```python
from build123d import *

# Parameters (mm, degrees)
F0_R     = 38.1
F1_DEPTH = 1778
F2_R     = 34.925
F3_DEPTH = 25.4
F4_R     = 34.925
F5_DEPTH = 25.4
F6_W     = 25.4
F6_H     = 25.4
F7_DEPTH = 38.1
F8_W     = 25.4
F8_H     = 25.4
F9_DEPTH = 38.1
F10_R    = 5.08
F11_R    = 5.08


# Not quite as in the source:
# - a pattern or mirror of a feature is missing from the dataset's text; its kind, count and spacing are read off the source's solid


with BuildPart() as f1:
    # F0 (on Front) → F1 (new body)
    with BuildSketch(Plane.XZ):
        Circle(F0_R)
    extrude(amount=F1_DEPTH)

    # F2 (on face) → F3 (join)
    with BuildSketch(Plane.XZ.offset(1778)):
        Circle(F2_R)
    extrude(amount=F3_DEPTH)

    # F4 (on face) → F5 (join)
    with BuildSketch(Plane(origin=(0, 0, 0), x_dir=(-1, 0, 0), z_dir=(0, 1, 0))):
        Circle(F4_R)
    extrude(amount=F5_DEPTH)

    # F6 (on face) → F7 (join)
    with BuildSketch(Plane.XZ.offset(1803.4)):
        Rectangle(F6_W, F6_H)
    f7 = extrude(amount=F7_DEPTH)

    # F7_copies: F7 across plane
    add(f7.mirror(Plane.ZX.offset(-882.65)))

    # F8 (on face) → F9 (join)
    with BuildSketch(Plane(origin=(0, 25.4, 0), x_dir=(-1, 0, 0), z_dir=(0, 1, 0))):
        Rectangle(F8_W, F8_H)
    extrude(amount=F9_DEPTH)

    # F10
    f10_edges = [f1.edges().sort_by_distance(p)[0] for p in [
        (34.925, 25.4, 0),
    ]]
    fillet(f10_edges, radius=F10_R)

    # F11
    f11_edges = [f1.edges().sort_by_distance(p)[0] for p in [
        (-34.925, -1803.4, 0),
    ]]
    fillet(f11_edges, radius=F11_R)


solid = f1.part
```
Check sheet for the modelled part. Datum: model origin and axes. Units: mm. A direction names the side the tool comes from. Round coordinates to 2 decimals unless told otherwise and drop trailing zeros. Write each loop counter-clockwise with the first axis right and the second up, starting at its lowest first coordinate (ties: lowest second). Pieces come first, ordered by that corner, then holes. Notation, with made-up numbers: (67, -39) -> (117, -39) arc R28 cw to (117, -1) -> close; hole circle Ø1 at (-39.75, 30). An arc over 180 degrees is marked (long way). Put each result on its own line as item: value.
(1) Sectioned sample at B-B (x = 0). Enter the section's corners in (y, z) (3 decimals), plus the area to 3 significant figures.
Values found:
outline: (-1841.5, -12.7) -> (-1803.4, -12.7) -> (-1803.4, -29.845) arc R5.08 ccw to (-1798.32, -34.925) -> (-1778, -34.925) -> (-1778, -38.1) -> (0, -38.1) -> (0, -34.925) -> (20.32, -34.925) arc R5.08 ccw to (25.4, -29.845) -> (25.4, -12.7) -> (76.2, -12.7) -> (76.2, 12.7) -> (25.4, 12.7) -> (25.4, 29.845) arc R5.08 ccw to (20.32, 34.925) -> (0, 34.925) -> (0, 38.1) -> (-1778, 38.1) -> (-1778, 34.925) -> (-1798.32, 34.925) arc R5.08 ccw to (-1803.4, 29.845) -> (-1803.4, 12.7) -> (-1841.5, 12.7) -> close
area: 141,000 mm^2
(2) Material ranges on line 1 (Y direction, x = 30.5, z = -4); line 2 (Y direction, x = -5, z = 25.5); line 3 (Z direction, x = 14.5, y = -247.5), recorded low to high.
Values found:
line 1: y = -1803.32 to 25.32
line 2: y = -1803.4 to 25.4
line 3: z = -35.23 to 35.23
(3) Sectioned sample at A-A (z = 0). Enter the section's corners in (x, y) (3 decimals).
Values found:
outline: (-38.1, -1778) -> (-34.925, -1778) -> (-34.925, -1798.32) arc R5.08 ccw to (-29.845, -1803.4) -> (-12.7, -1803.4) -> (-12.7, -1841.5) -> (12.7, -1841.5) -> (12.7, -1803.4) -> (29.845, -1803.4) arc R5.08 ccw to (34.925, -1798.32) -> (34.925, -1778) -> (38.1, -1778) -> (38.1, 0) -> (34.925, 0) -> (34.925, 20.32) arc R5.08 ccw to (29.845, 25.4) -> (12.7, 25.4) -> (12.7, 76.2) -> (-12.7, 76.2) -> (-12.7, 25.4) -> (-29.845, 25.4) arc R5.08 ccw to (-34.925, 20.32) -> (-34.925, 0) -> (-38.1, 0) -> close
(4) Go/stop test with flat-tipped pins: pin 1 Ø12.5 at (y, z) = (53.5, 2) entering from +X; pin 2 Ø20.5 at (x, y) = (3.5, 51) entering from -Z; pin 3 Ø7.5 at (x, y) = (0, -1822) entering from +Z; pin 4 Ø4 at (x, z) = (14.5, 8.5) entering from +Y. Record where each tip stops, or that it passes through.
Values found:
pin 1: stops at x = 12.7
pin 2: stops at z = -12.7
pin 3: stops at z = 12.7
pin 4: stops at y = 76.2
(5) Tool access check on faces 1 (the face through (-27.715, -1788.018, -21.251)), 2 (the face through (17, 0, -31)), 3 (the face through (-30.235, -876.554, -23.183)). Record the directions out of +Z, -Z, +X, -X, +Y, -Y that give a thin tool (end or side, any length) a straight path to the whole face; none if there is none.
Values found:
face 1: -Y
face 2: +Y
face 3: +Y, -Y
(6) Sectioned sample at C-C (y = -538.5). Enter the section's corners in (x, z), plus the area to 3 significant figures.
Values found:
outline: circle Ø76.2 at (0, 0)
area: 4,560 mm^2
